```python
from build123d import *

# Parameters (mm, degrees)
BOSS_EXTRUDE2_DEPTH   = 2.8
BOSS_EXTRUDE2_2_DEPTH = 2.8
BOSS_EXTRUDE1_START   = 3
BOSS_EXTRUDE1_DEPTH   = 3
FILLET1_R             = 1


with BuildPart() as part:
    # Sketch3 → Boss-Extrude2 (new body)
    with BuildSketch(Plane.XY):
        with BuildLine():
            Line((25.75, 5.75), (27.75, 5.75))
            Line((27.75, 5.75), (27.75, 7.75))
            ThreePointArc((27.75, 7.75), (27.457106781, 8.457106781), (26.75, 8.75))
            Line((26.75, 8.75), (-26.75, 8.75))
            ThreePointArc((-26.75, 8.75), (-27.457106781, 8.457106781), (-27.75, 7.75))
            Line((-27.75, 7.75), (-27.75, 5.75))
            Line((-27.75, 5.75), (-25.75, 5.75))
            Line((-25.75, 5.75), (-25.75, 6.75))
            Line((-25.75, 6.75), (25.75, 6.75))
            Line((25.75, 6.75), (25.75, 5.75))
        make_face()
    extrude(amount=-BOSS_EXTRUDE2_DEPTH)



with BuildPart() as body_2:
    # Sketch3 → Boss-Extrude2 2 (new body)
    with BuildSketch(Plane.XY):
        with BuildLine():
            Line((-25.75, -6.75), (-25.75, -5.75))
            Line((-25.75, -5.75), (-27.75, -5.75))
            Line((-27.75, -5.75), (-27.75, -7.75))
            ThreePointArc((-27.75, -7.75), (-27.457106781, -8.457106781), (-26.75, -8.75))
            Line((-26.75, -8.75), (26.75, -8.75))
            ThreePointArc((26.75, -8.75), (27.457106781, -8.457106781), (27.75, -7.75))
            Line((27.75, -7.75), (27.75, -5.75))
            Line((27.75, -5.75), (25.75, -5.75))
            Line((25.75, -5.75), (25.75, -6.75))
            Line((25.75, -6.75), (-25.75, -6.75))
        make_face()
    extrude(amount=-BOSS_EXTRUDE2_2_DEPTH)


with BuildPart() as part_1:
    add(part.part)

    add(body_2.part)  # Boss-Extrude1 merges body 2
    # Sketch2 → Boss-Extrude1 (add)
    with BuildSketch(Plane.XY.offset(BOSS_EXTRUDE1_START)):
        with BuildLine():
            Line((24.25, 5.75), (27.75, 5.75))
            Line((27.75, 5.75), (27.75, 7.75))
            ThreePointArc((27.75, 7.75), (27.457106781, 8.457106781), (26.75, 8.75))
            Line((26.75, 8.75), (-26.75, 8.75))
            ThreePointArc((-26.75, 8.75), (-27.457106781, 8.457106781), (-27.75, 7.75))
            Line((-27.75, 7.75), (-27.75, 5.75))
            Line((-27.75, 5.75), (-24.25, 5.75))
            Line((-24.25, 5.75), (-24.25, -5.75))
            Line((-24.25, -5.75), (-27.75, -5.75))
            Line((-27.75, -5.75), (-27.75, -7.75))
            ThreePointArc((-27.75, -7.75), (-27.457106781, -8.457106781), (-26.75, -8.75))
            Line((-26.75, -8.75), (26.75, -8.75))
            ThreePointArc((26.75, -8.75), (27.457106781, -8.457106781), (27.75, -7.75))
            Line((27.75, -7.75), (27.75, -5.75))
            Line((27.75, -5.75), (24.25, -5.75))
            Line((24.25, -5.75), (24.25, 5.75))
        make_face()
        with BuildLine():
            ThreePointArc((30.75, 10.75), (30.457106781, 11.457106781), (29.75, 11.75))
            Line((29.75, 11.75), (-29.75, 11.75))
            ThreePointArc((-29.75, 11.75), (-30.457106781, 11.457106781), (-30.75, 10.75))
            Line((-30.75, 10.75), (-30.75, 5.75))
            Line((-30.75, 5.75), (-27.75, 5.75))
            Line((-27.75, 5.75), (-27.75, 7.75))
            ThreePointArc((-27.75, 7.75), (-27.457106781, 8.457106781), (-26.75, 8.75))
            Line((-26.75, 8.75), (26.75, 8.75))
            ThreePointArc((26.75, 8.75), (27.457106781, 8.457106781), (27.75, 7.75))
            Line((27.75, 7.75), (27.75, 5.75))
            Line((27.75, 5.75), (30.75, 5.75))
            Line((30.75, 5.75), (30.75, 10.75))
        make_face()
        with BuildLine():
            Line((-30.75, -5.75), (-30.75, -10.75))
            ThreePointArc((-30.75, -10.75), (-30.457106781, -11.457106781), (-29.75, -11.75))
            Line((-29.75, -11.75), (29.75, -11.75))
            ThreePointArc((29.75, -11.75), (30.457106781, -11.457106781), (30.75, -10.75))
            Line((30.75, -10.75), (30.75, -5.75))
            Line((30.75, -5.75), (27.75, -5.75))
            Line((27.75, -5.75), (27.75, -7.75))
            ThreePointArc((27.75, -7.75), (27.457106781, -8.457106781), (26.75, -8.75))
            Line((26.75, -8.75), (-26.75, -8.75))
            ThreePointArc((-26.75, -8.75), (-27.457106781, -8.457106781), (-27.75, -7.75))
            Line((-27.75, -7.75), (-27.75, -5.75))
            Line((-27.75, -5.75), (-30.75, -5.75))
        make_face()
    extrude(amount=-BOSS_EXTRUDE1_DEPTH)

    # Fillet1
    fillet1_edges = [part_1.edges().sort_by_distance(p)[0] for p in [
        (24.25, -5.75, 1.5),
        (24.25, 5.75, 1.5),
        (-24.25, -5.75, 1.5),
        (-24.25, 5.75, 1.5),
        (-24.25, 0, 3),
        (-27.5, 5.75, 3),
        (-30.75, 8.25, 3),
        (-30.457106781, 11.457106781, 3),
        (0, 11.75, 3),
        (30.457106781, 11.457106781, 3),
        (30.75, 8.25, 3),
        (27.5, 5.75, 3),
        (24.25, 0, 3),
        (27.5, -5.75, 3),
        (30.75, -8.25, 3),
        (30.457106781, -11.457106781, 3),
        (0, -11.75, 3),
        (-30.457106781, -11.457106781, 3),
        (-30.75, -8.25, 3),
        (-27.5, -5.75, 3),
        (0, 6.75, 0),
        (0, -6.75, 0),
    ]]
    fillet(fillet1_edges, radius=FILLET1_R - 0.0001)  # a hair under: the kernel refuses the full size


solid = part_1.part
```
Verification items for the finished model (mm, model axes). A direction names the side the tool comes from. Round coordinates to 2 decimals unless told otherwise and drop trailing zeros. Order: outer loops, then holes, each group sorted by start corner. A loop starts at its lowest first (then second) coordinate and runs counter-clockwise, first axis right, second up. Notation, with made-up numbers: (15, 89.25) - (29, 89.25) arc R26 ccw to (29, 103.25) - close; hole circle Ø3 at (8, 82). An arc over 180 degrees is marked (long way). Use CSV: the item, a comma, the result in double quotes.
(1) Section check C-C on z = 0.65. Record the boundary of the cut face in (x, y).
Entries:
outline,"(-30.75, -10.75) arc R1 ccw to (-29.75, -11.75) - (29.75, -11.75) arc R1 ccw to (30.75, -10.75) - (30.75, -5.75) - (25.25, -5.75) arc R1 cw to (24.25, -4.75) - (24.25, 4.75) arc R1 cw to (25.25, 5.75) - (30.75, 5.75) - (30.75, 10.75) arc R1 ccw to (29.75, 11.75) - (-29.75, 11.75) arc R1 ccw to (-30.75, 10.75) - (-30.75, 5.75) - (-25.25, 5.75) arc R1 cw to (-24.25, 4.75) - (-24.25, -4.75) arc R1 cw to (-25.25, -5.75) - (-30.75, -5.75) - close"
(2) Mould release check, pull along X, two halves, no side actions. Record for faces 6 (the face through (-24.551, 5.465, 0.986)), 7 (the face through (30.75, 8, 1)), 8 (the face through (25.75, -6, -1)): released by +X, released by -X, zero draft, split by the parting line, or undercut.
Entries:
face 6,"released by -X"
face 7,"released by +X"
face 8,"undercut"
(3) Section check B-B on x = 11. Record the boundary of the cut face in (y, z), and give its area (3 significant figures).
Entries:
outline,"(-11.75, 0) - (-8.75, 0) - (-8.75, -2.8) - (-6.75, -2.8) - (-6.75, -1) arc R1 cw to (-5.75, 0) - (5.75, 0) arc R1 cw to (6.75, -1) - (6.75, -2.8) - (8.75, -2.8) - (8.75, 0) - (11.75, 0) - (11.75, 2) arc R1 ccw to (10.75, 3) - (-10.75, 3) arc R1 ccw to (-11.75, 2) - close"
area,"81.7 mm^2"
(4) Gauge pin test, flat ends, axial feed: pin 1 Ø0.8 at (y, z) = (6.5, -1) entering from -X; pin 2 Ø9 at (x, y) = (-10, 2) entering from -Z; pin 3 Ø1.6 at (y, z) = (7, -1) entering from +X; pin 4 Ø1.4 at (x, z) = (28.5, -1) entering from +Y. Record the tip position at first contact, or that the pin passes through.
Entries:
pin 1,"x = -27.75"
pin 2,"z = -0.34"
pin 3,"x = 27.75"
pin 4,"through"
(5) Section check A-A on z = -1.9. Record the boundary of the cut face in (x, y).
Entries:
outline,"(-27.75, -7.75) arc R1 ccw to (-26.75, -8.75) - (26.75, -8.75) arc R1 ccw to (27.75, -7.75) - (27.75, -5.75) - (25.75, -5.75) - (25.75, -6.75) - (-25.75, -6.75) - (-25.75, -5.75) - (-27.75, -5.75) - close; (-27.75, 5.75) - (-25.75, 5.75) - (-25.75, 6.75) - (25.75, 6.75) - (25.75, 5.75) - (27.75, 5.75) - (27.75, 7.75) arc R1 ccw to (26.75, 8.75) - (-26.75, 8.75) arc R1 ccw to (-27.75, 7.75) - close"
(6) Thickness scan on probe 1 along Y at (x, z) = (-6, -0.95); probe 2 along Y at (x, z) = (26, -0.9); probe 3 along X at (y, z) = (6, -2.25). Record the ranges inside material, lowest first. Write a range as from..to.
Entries:
probe 1,"-8.75..-6.75, 6.75..8.75"
probe 2,"-8.75..-5.75, 5.75..8.75"
probe 3,"-27.75..-25.75, 25.75..27.75"
(7) Access from +Z, -Z, +X, -X, +Y, -Y to the whole of each face (thin tool, end or side, straight path). Record for faces 1 (the face through (-27.449, 8.465, -1.38)), 2 (the face through (-27.75, -7, -1)), 3 (the face through (-25.75, 6, -1)), 4 (the face through (-27, 5.75, 0)), 5 (the face through (27, 5.75, 0)).
Entries:
face 1,"-Z, -X, +Y"
face 2,"-Z, -X, +Y, -Y"
face 3,"-Z"
face 4,"+Z, -Z, -X"
face 5,"+Z, -Z, +X"
(8) Section check D-D on y = -2. Record the boundary of the cut face in (x, z), and give its area (3 significant figures).
Entries:
outline,"(-24.25, 0) - (24.25, 0) - (24.25, 2) arc R1 ccw to (23.25, 3) - (-23.25, 3) arc R1 ccw to (-24.25, 2) - close"
area,"145 mm^2"
